For this review, take the finished solid that the model builds, in its own axes (mm). A direction names the side the tool comes from. Coordinates: 2 decimals unless noted, no trailing zeros. Loops run counter-clockwise (first coordinate to the right, second up) from the corner with the lowest first, then second, coordinate; pieces in that order, holes last. Notation, with made-up numbers: M 0,-18.75 L 14,-18.75 A22 cw 14,20.25 Z; hole C 69,-24.75 d2. An arc over 180 degrees is marked long. Put each result on its own line as item: value.
```python
from build123d import *

# Parameters (mm, degrees)
F0_R     = 9.525
F0_R_2   = 5
F1_DEPTH = 25.4
F2_DEPTH = 12.7
F4_D     = 8.8
F4_DEPTH = 19.05
F4_TIP   = 2.6437867237


with BuildPart() as f1:
    # F0 (on Top) → F1 (new body)
    with BuildSketch(Plane.XY):
        Circle(F0_R)
        Circle(F0_R_2, mode=Mode.SUBTRACT)
        Circle(F0_R_2)
    extrude(amount=F1_DEPTH)

    # F0 (on Top) → F2 (join)
    with BuildSketch(Plane.XY):
        Circle(F0_R_2)
    extrude(amount=-F2_DEPTH)

    # F4
    with Locations(Plane.XY.offset(25.4)):
        with Locations((0, 0)):
            Hole(F4_D / 2, depth=F4_DEPTH)
            with Locations((0, 0, -(F4_DEPTH + F4_TIP / 2))):  # 118° drill point
                Cone(0, F4_D / 2, F4_TIP, mode=Mode.SUBTRACT)


solid = f1.part
```
(1) For pin 1 (4 mm diameter, centred on y = -2, z = -7, fed in from -X); pin 2 (1.5 mm diameter, centred on x = 5, z = 1.5, fed in from -Y); pin 3 (1 mm diameter, centred on x = -3, y = 7, fed in from -Z), all flat-tipped, find the tip position at first contact; note any pin that passes through.
Determined:
pin 1: stops at x = -5
pin 2: stops at y = -8.52
pin 3: stops at z = 0
(2) Wall thickness on line 1 along Y through (x, z) = (0, 17.5) (3 decimals); line 2 along Z through (x, y) = (-7.25, 5.5); line 3 along X through (y, z) = (0.25, -4.5): over which ranges is each line inside the solid? List them lowest first. Write a range as [from, to].
Determined:
line 1: y = [-9.525, -4.4], [4.4, 9.525]
line 2: z = [0, 25.4]
line 3: x = [-4.99, 4.99]
(3) Add section C-C (x = -6.5). Write out the cut boundary in (y, z), plus the area to 3 significant figures.
Determined:
outline: M -6.96,0 L 6.96,0 L 6.96,25.4 L -6.96,25.4 Z
area: 354 mm^2
(4) Add section A-A (z = 20.5). Write out the cut boundary in (x, y) (3 decimals).
Determined:
outline: C 0,0 d19.05; hole C 0,0 d8.8
(5) Add section B-B (z = -3.5). Write out the cut boundary in (x, y).
Determined:
outline: C 0,0 d10
(6) Tool access review of faces 1 (the conical face through (0.729, 0.23, 4.165)), 2 (the flat face through (4, -4, 0)): name each direction out of +Z, -Z, +X, -X, +Y, -Y from which nothing blocks a thin tool from reaching the whole face with its end or side.
Determined:
face 1: +Z
face 2: -Z
(7) Draft analysis for pull direction X (two halves, no side actions). For faces 3 (the flat face through (0, 0, -12.7)), 4 (the cylindrical face through (-4.197, 1.322, 15.742)), 5 (the cylindrical face through (-1.08, -4.88, -6.26)), state which applies: +X half, -X half, draft (parallel to the pull), parting line (faces both ways), or undercut.
Determined:
face 3: draft
face 4: undercut
face 5: parting line
